Source: CAD feature listing. Evaluate the final solid. Frame: model axes, mm. A direction names the side the tool comes from. Give positions to 0.01 mm unless a question says otherwise; leave off trailing zeros. Order: outer loops, then holes, each group sorted by start corner. A loop starts at its lowest first (then second) coordinate and runs counter-clockwise, first axis right, second up.
from build123d import *

# Parameters (mm, degrees)
F0_W     = 50.8
F0_H     = 38.1
F0_R     = 9.525
F1_DEPTH = 88.9
F2_DEPTH = 25.4
F3_DEPTH = 12.7


with BuildPart() as f1:
    # F0 (on Top) → F1 (new body)
    with BuildSketch(Plane.XY):
        with Locations((25.4, 95.25)):
            Rectangle(F0_W, F0_H)
        with Locations((25.4, 57.15)):
            Rectangle(F0_W, F0_H)
        with Locations((25.4, 57.15)):
            Circle(F0_R, mode=Mode.SUBTRACT)
        with Locations((25.4, 19.05)):
            Rectangle(F0_W, F0_H)
        Polygon((101.6, 114.3), (50.8, 114.3), (50.8, 76.2), (50.8, 38.1), (50.8, 0), (101.6, 0), (101.6, 38.1), (101.6, 76.2), align=None)
        Polygon((152.4, 114.3), (101.6, 114.3), (101.6, 76.2), (169.3333333333, 76.2), align=None)
        Polygon((169.3333333333, 76.2), (101.6, 76.2), (101.6, 38.1), (169.3333333333, 38.1), (177.8, 57.15), align=None)
        with Locations((127, 57.15)):
            Circle(F0_R, mode=Mode.SUBTRACT)
        Polygon((169.3333333333, 38.1), (101.6, 38.1), (101.6, 0), (152.4, 0), align=None)
    extrude(amount=-F1_DEPTH)

    # F0 (on Top) → F2 (join)
    with BuildSketch(Plane.XY):
        with Locations((25.4, 95.25)):
            Rectangle(F0_W, F0_H)
        with Locations((25.4, 19.05)):
            Rectangle(F0_W, F0_H)
        Polygon((152.4, 114.3), (101.6, 114.3), (101.6, 76.2), (169.3333333333, 76.2), align=None)
        Polygon((169.3333333333, 38.1), (101.6, 38.1), (101.6, 0), (152.4, 0), align=None)
    extrude(amount=F2_DEPTH)

    # F0 (on Top) → F3 (join)
    with BuildSketch(Plane.XY):
        with Locations((25.4, 57.15)):
            Rectangle(F0_W, F0_H)
        with Locations((25.4, 57.15)):
            Circle(F0_R, mode=Mode.SUBTRACT)
        Polygon((169.3333333333, 76.2), (101.6, 76.2), (101.6, 38.1), (169.3333333333, 38.1), (177.8, 57.15), align=None)
        with Locations((127, 57.15)):
            Circle(F0_R, mode=Mode.SUBTRACT)
    extrude(amount=F3_DEPTH)


solid = f1.part
(1) Pin query (flat end, axial travel): pin 1 Ø12.5 at (y, z) = (72, 14) entering from +X; pin 2 Ø20.5 at (y, z) = (44.5, 11.5) entering from -X; pin 3 Ø15 at (x, y) = (78.5, 59.5) entering from +Z; pin 4 Ø25 at (x, y) = (127, 57.15) entering from +Z. Return the tip coordinate at first contact, or that it passes through.
(2) Section D-D, the plane x = 154.5. Return loops of the section in (y, z) (3 decimals), plus the area to 3 significant figures.
(3) Section B-B, the plane y = 45. Return loops of the section in (x, z), plus the area to 3 significant figures.
(4) Draft query along Y for faces 4 (the flat face through (127, 19, 25.4)), 5 (the flat face through (75, 0, -31)), 6 (the flat face through (25, 38.1, 19)). Return one class per face: +Y half, -Y half, draft (parallel to the pull), parting line (faces both ways), or undercut.
(5) Section C-C, the plane z = -19. Return loops of the section in (x, y) (3 decimals).
(6) Line query: line 1 along Y through (x, z) = (127, -59.5) (3 decimals); line 2 along Y through (x, z) = (122, 18); line 3 along Z through (x, y) = (117, 63.5). Output: solid intervals per line, ascending.
(7) Section A-A, the plane x = 127. Return loops of the section in (y, z) (3 decimals).
(8) Access query for faces 1 (the flat face through (25, 96, 25.4)), 2 (the flat face through (135, 76.2, 19)), 3 (the flat face through (50.8, 56.3, 12.5)). Directions: +Z, -Z, +X, -X, +Y, -Y. A direction counts if a zero-diameter tool reaches every point of the face in a straight line with its end or side. Return the directions, or none.
Checks:
1. pin 1: stops at x = 173.92
1. pin 2: stops at x = 0
1. pin 3: stops at z = 0
1. pin 4: stops at z = 12.7
2. outline: (4.725, -88.9) - (109.575, -88.9) - (109.575, 25.4) - (76.2, 25.4) - (76.2, 12.7) - (38.1, 12.7) - (38.1, 25.4) - (4.725, 25.4) - close
2. area: 11,500 mm2
3. outline: (0, -88.9) - (172.4, -88.9) - (172.4, 12.7) - (101.6, 12.7) - (101.6, 0) - (50.8, 0) - (50.8, 12.7) - (0, 12.7) - close
3. area: 16,900 mm2
4. face 4: draft
4. face 5: -Y half
4. face 6: undercut
5. outline: (0, 0) - (152.4, 0) - (177.8, 57.15) - (152.4, 114.3) - (0, 114.3) - close; hole circle Ø19.05 at (25.4, 57.15); hole circle Ø19.05 at (127, 57.15)
6. line 1: y = 0 to 47.625, 66.675 to 114.3
6. line 2: y = 0 to 38.1, 76.2 to 114.3
6. line 3: z = -88.9 to 12.7
7. outline: (0, -88.9) - (47.625, -88.9) - (47.625, 12.7) - (38.1, 12.7) - (38.1, 25.4) - (0, 25.4) - close; (66.675, -88.9) - (114.3, -88.9) - (114.3, 25.4) - (76.2, 25.4) - (76.2, 12.7) - (66.675, 12.7) - close
8. face 1: +Z, +X, -X, +Y, -Y
8. face 2: +Z, +X, -X
8. face 3: +Z, +Y, -Y
